Read the model definition and answer for the solid it produces. Units are mm, in the model's axes. Give positions to 0.01 mm unless a question says otherwise; leave off trailing zeros. Order: outer loops, then holes, each group sorted by start corner. A loop starts at its lowest first (then second) coordinate and runs counter-clockwise, first axis right, second up. Notation, with made-up numbers: (51, 39) - (82, 39) arc R13 ccw to (82, 55) - close; hole circle Ø9 at (56, 0). An arc over 180 degrees is marked (long way). Use a Markdown table: item, result. Add a question column.
1. Consider L1, parallel to X at y = 171, z = 9; L2, parallel to X at y = 271.5, z = 3.25; L3, parallel to Y at x = 145.5, z = 1.75. Determine where each line is inside the solid, lowest interval first.
2. A cutting plane is placed at A-A on y = 168. Determine the outline of the cut face in (x, z), and give its area (3 significant figures).
3. A cutting plane is placed at C-C on z = 1.5. State how many separate pieces and enclosed holes the cut face has, and give its area (3 significant figures).
4. Flat-ended cylindrical pins translate along their axes: P1, Ø3, axis at y = -192.5, z = 3, coming from the +X side; P2, Ø5, axis at x = -100, z = 5.5, coming from the -Y side; P3, Ø5, axis at x = 72, z = 3.5, coming from the +Y side; P4, Ø5, axis at x = 17, y = -29.5, coming from the -Z side. Find the tip coordinate at first contact, or state that the pin passes through.
5. A cutting plane is placed at B-B on y = 279. Determine the outline of the cut face in (x, z).
```python
from build123d import *

# Parameters (mm, degrees)
BOSS_EXTRU_1_DEPTH      = 10
ESQUISSE2_W             = 150
ESQUISSE2_H             = 120
BOSS_EXTRU_2_DEPTH      = 10
ESQUISSE3_W             = 10
ESQUISSE3_H             = 50
ESQUISSE3_W_2           = 50
ESQUISSE3_H_2           = 10
ENL_V_MAT_EXTRU_1_DEPTH = 10
ESQUISSE4_W             = 50
ESQUISSE4_H             = 10
ENL_V_MAT_EXTRU_2_DEPTH = 10


with BuildPart() as part:
    # Esquisse1 → Boss.-Extru.1 (new body)
    with BuildSketch(Plane.XY):
        Polygon((-50, 335.901139535), (50, 335.901139535), (255.775862069, 10.507079064), (205, -75.642859016), (-205, -75.642859016), (-255.775862069, 10.507079064), align=None)
        with BuildLine():
            Line((-189.319805153, 31.819805153), (-191.794678888, 34.294678888))
            ThreePointArc((-191.794678888, 34.294678888), (-206, 0), (-191.794678888, -34.294678888))
            Line((-191.794678888, -34.294678888), (-189.319805153, -31.819805153))
            ThreePointArc((-189.319805153, -31.819805153), (-202.5, 0), (-189.319805153, 31.819805153))
        make_face(mode=Mode.SUBTRACT)
        with BuildLine():
            Line((-125.680194847, 31.819805153), (-123.205321112, 34.294678888))
            ThreePointArc((-123.205321112, 34.294678888), (-109, 0), (-123.205321112, -34.294678888))
            Line((-123.205321112, -34.294678888), (-125.680194847, -31.819805153))
            ThreePointArc((-125.680194847, -31.819805153), (-112.5, 0), (-125.680194847, 31.819805153))
        make_face(mode=Mode.SUBTRACT)
        with BuildLine():
            Line((-84.319805153, -31.819805153), (-86.794678888, -34.294678888))
            ThreePointArc((-86.794678888, -34.294678888), (-101, 0), (-86.794678888, 34.294678888))
            Line((-86.794678888, 34.294678888), (-84.319805153, 31.819805153))
            ThreePointArc((-84.319805153, 31.819805153), (-97.5, 0), (-84.319805153, -31.819805153))
        make_face(mode=Mode.SUBTRACT)
        with BuildLine():
            Line((-20.680194847, 31.819805153), (-18.205321112, 34.294678888))
            ThreePointArc((-18.205321112, 34.294678888), (-4, 0), (-18.205321112, -34.294678888))
            Line((-18.205321112, -34.294678888), (-20.680194847, -31.819805153))
            ThreePointArc((-20.680194847, -31.819805153), (-7.5, 0), (-20.680194847, 31.819805153))
        make_face(mode=Mode.SUBTRACT)
        with BuildLine():
            Line((20.680194847, -31.819805153), (18.205321112, -34.294678888))
            ThreePointArc((18.205321112, -34.294678888), (4, 0), (18.205321112, 34.294678888))
            Line((18.205321112, 34.294678888), (20.680194847, 31.819805153))
            ThreePointArc((20.680194847, 31.819805153), (7.5, 0), (20.680194847, -31.819805153))
        make_face(mode=Mode.SUBTRACT)
        with BuildLine():
            Line((84.319805153, 31.819805153), (86.794678888, 34.294678888))
            ThreePointArc((86.794678888, 34.294678888), (101, 0), (86.794678888, -34.294678888))
            Line((86.794678888, -34.294678888), (84.319805153, -31.819805153))
            ThreePointArc((84.319805153, -31.819805153), (97.5, 0), (84.319805153, 31.819805153))
        make_face(mode=Mode.SUBTRACT)
        with BuildLine():
            Line((125.680194847, -31.819805153), (123.205321112, -34.294678888))
            ThreePointArc((123.205321112, -34.294678888), (109, 0), (123.205321112, 34.294678888))
            Line((123.205321112, 34.294678888), (125.680194847, 31.819805153))
            ThreePointArc((125.680194847, 31.819805153), (112.5, 0), (125.680194847, -31.819805153))
        make_face(mode=Mode.SUBTRACT)
        with BuildLine():
            Line((189.319805153, 31.819805153), (191.794678888, 34.294678888))
            ThreePointArc((191.794678888, 34.294678888), (206, 0), (191.794678888, -34.294678888))
            Line((191.794678888, -34.294678888), (189.319805153, -31.819805153))
            ThreePointArc((189.319805153, -31.819805153), (202.5, 0), (189.319805153, 31.819805153))
        make_face(mode=Mode.SUBTRACT)
        with BuildLine():
            Line((-139.294678888, 56.63798851), (-136.819805153, 59.112862244))
            ThreePointArc((-136.819805153, 59.112862244), (-150, 90.932667397), (-136.819805153, 122.752472551))
            Line((-136.819805153, 122.752472551), (-139.294678888, 125.227346285))
            ThreePointArc((-139.294678888, 125.227346285), (-153.5, 90.932667397), (-139.294678888, 56.63798851))
        make_face(mode=Mode.SUBTRACT)
        with BuildLine():
            Line((-70.705321112, 56.63798851), (-73.180194847, 59.112862244))
            ThreePointArc((-73.180194847, 59.112862244), (-60, 90.932667397), (-73.180194847, 122.752472551))
            Line((-73.180194847, 122.752472551), (-70.705321112, 125.227346285))
            ThreePointArc((-70.705321112, 125.227346285), (-56.5, 90.932667397), (-70.705321112, 56.63798851))
        make_face(mode=Mode.SUBTRACT)
        with BuildLine():
            Line((-31.819805153, 122.752472551), (-34.294678888, 125.227346285))
            ThreePointArc((-34.294678888, 125.227346285), (-48.5, 90.932667397), (-34.294678888, 56.63798851))
            Line((-34.294678888, 56.63798851), (-31.819805153, 59.112862244))
            ThreePointArc((-31.819805153, 59.112862244), (-45, 90.932667397), (-31.819805153, 122.752472551))
        make_face(mode=Mode.SUBTRACT)
        with BuildLine():
            Line((34.294678888, 56.63798851), (31.819805153, 59.112862244))
            ThreePointArc((31.819805153, 59.112862244), (45, 90.932667397), (31.819805153, 122.752472551))
            Line((31.819805153, 122.752472551), (34.294678888, 125.227346285))
            ThreePointArc((34.294678888, 125.227346285), (48.5, 90.932667397), (34.294678888, 56.63798851))
        make_face(mode=Mode.SUBTRACT)
        with BuildLine():
            Line((73.180194847, 122.752472551), (70.705321112, 125.227346285))
            ThreePointArc((70.705321112, 125.227346285), (56.5, 90.932667397), (70.705321112, 56.63798851))
            Line((70.705321112, 56.63798851), (73.180194847, 59.112862244))
            ThreePointArc((73.180194847, 59.112862244), (60, 90.932667397), (73.180194847, 122.752472551))
        make_face(mode=Mode.SUBTRACT)
        with BuildLine():
            Line((139.294678888, 56.63798851), (136.819805153, 59.112862244))
            ThreePointArc((136.819805153, 59.112862244), (150, 90.932667397), (136.819805153, 122.752472551))
            Line((136.819805153, 122.752472551), (139.294678888, 125.227346285))
            ThreePointArc((139.294678888, 125.227346285), (153.5, 90.932667397), (139.294678888, 56.63798851))
        make_face(mode=Mode.SUBTRACT)
        with BuildLine():
            Line((-84.319805153, 213.685139948), (-86.794678888, 216.160013682))
            ThreePointArc((-86.794678888, 216.160013682), (-101, 181.865334795), (-86.794678888, 147.570655907))
            Line((-86.794678888, 147.570655907), (-84.319805153, 150.045529641))
            ThreePointArc((-84.319805153, 150.045529641), (-97.5, 181.865334795), (-84.319805153, 213.685139948))
        make_face(mode=Mode.SUBTRACT)
        with BuildLine():
            Line((-20.680194847, 213.685139948), (-18.205321112, 216.160013682))
            ThreePointArc((-18.205321112, 216.160013682), (-4, 181.865334795), (-18.205321112, 147.570655907))
            Line((-18.205321112, 147.570655907), (-20.680194847, 150.045529641))
            ThreePointArc((-20.680194847, 150.045529641), (-7.5, 181.865334795), (-20.680194847, 213.685139948))
        make_face(mode=Mode.SUBTRACT)
        with BuildLine():
            Line((20.680194847, 150.045529641), (18.205321112, 147.570655907))
            ThreePointArc((18.205321112, 147.570655907), (4, 181.865334795), (18.205321112, 216.160013682))
            Line((18.205321112, 216.160013682), (20.680194847, 213.685139948))
            ThreePointArc((20.680194847, 213.685139948), (7.5, 181.865334795), (20.680194847, 150.045529641))
        make_face(mode=Mode.SUBTRACT)
        with BuildLine():
            Line((84.319805153, 150.045529641), (86.794678888, 147.570655907))
            ThreePointArc((86.794678888, 147.570655907), (101, 181.865334795), (86.794678888, 216.160013682))
            Line((86.794678888, 216.160013682), (84.319805153, 213.685139948))
            ThreePointArc((84.319805153, 213.685139948), (97.5, 181.865334795), (84.319805153, 150.045529641))
        make_face(mode=Mode.SUBTRACT)
        with BuildLine():
            Line((-31.819805153, 304.617807345), (-34.294678888, 307.09268108))
            ThreePointArc((-34.294678888, 307.09268108), (-48.5, 272.798002192), (-34.294678888, 238.503323305))
            Line((-34.294678888, 238.503323305), (-31.819805153, 240.978197039))
            ThreePointArc((-31.819805153, 240.978197039), (-45, 272.798002192), (-31.819805153, 304.617807345))
        make_face(mode=Mode.SUBTRACT)
        with BuildLine():
            Line((31.819805153, 304.617807345), (34.294678888, 307.09268108))
            ThreePointArc((34.294678888, 307.09268108), (48.5, 272.798002192), (34.294678888, 238.503323305))
            Line((34.294678888, 238.503323305), (31.819805153, 240.978197039))
            ThreePointArc((31.819805153, 240.978197039), (45, 272.798002192), (31.819805153, 304.617807345))
        make_face(mode=Mode.SUBTRACT)
    extrude(amount=BOSS_EXTRU_1_DEPTH)

    # Esquisse2 → Boss.-Extru.2 (add)
    with BuildSketch(Plane.XY.offset(10)):
        with Locations((0, -135.642859016)):
            Rectangle(ESQUISSE2_W, ESQUISSE2_H)
    extrude(amount=-BOSS_EXTRU_2_DEPTH)

    # Esquisse3 → Enlèv. mat.-Extru.1 (cut)
    with BuildSketch(Plane.XY.offset(10)):
        with Locations((-70, -135.642859016)):
            Rectangle(ESQUISSE3_W, ESQUISSE3_H)
        with Locations((0, -190.642859016)):
            Rectangle(ESQUISSE3_W_2, ESQUISSE3_H_2)
        with Locations((70, -135.642859016)):
            Rectangle(ESQUISSE3_W, ESQUISSE3_H)
    extrude(amount=-ENL_V_MAT_EXTRU_1_DEPTH, mode=Mode.SUBTRACT)

    # Esquisse4 → Enlèv. mat.-Extru.2 (cut)
    with BuildSketch(Plane.XY.offset(10)):
        with Locations((-140, -70.642859016)):
            Rectangle(ESQUISSE4_W, ESQUISSE4_H)
        Polygon((-217.693965517, -54.105374496), (-209.078971709, -49.027788289), (-234.466902744, -5.952819249), (-243.081896552, -11.030405456), align=None)
        Polygon((-229.051724138, 52.766047956), (-220.599930359, 47.42122037), (-167.151654497, 131.939158154), (-175.603448276, 137.283985741), align=None)
        Polygon((-68.272344153, 288.297343056), (-76.724137931, 293.642170642), (-130.172413793, 209.124232858), (-121.720620015, 203.779405271), align=None)
        with Locations((0, 330.901139535)):
            Rectangle(ESQUISSE4_W, ESQUISSE4_H)
        with Locations((140, -70.642859016)):
            Rectangle(ESQUISSE4_W, ESQUISSE4_H)
        Polygon((234.466902744, -5.952819249), (243.081896552, -11.030405456), (217.693965517, -54.105374496), (209.078971709, -49.027788289), align=None)
        Polygon((167.151654497, 131.939158154), (175.603448276, 137.283985741), (229.051724138, 52.766047956), (220.599930359, 47.42122037), align=None)
        Polygon((121.720620015, 203.779405271), (130.172413793, 209.124232858), (76.724137931, 293.642170642), (68.272344153, 288.297343056), align=None)
    extrude(amount=-ENL_V_MAT_EXTRU_2_DEPTH, mode=Mode.SUBTRACT)


solid = part.part
```
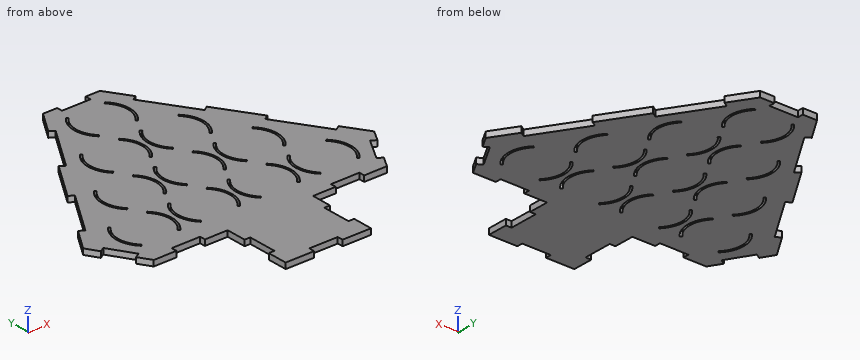
Output values:
| question | item | result |
|---|---|---|
| 1 | L1 | -154.28 to -99.77, -96.17 to -8.83, -5.23 to 5.23, 8.83 to 96.17, 99.77 to 154.28 |
| 1 | L2 | -78.89 to -48.48, -44.98 to 44.98, 48.48 to 78.89 |
| 1 | L3 | -65.64 to 64.25, 71.32 to 110.55, 117.62 to 184.89 |
| 2 | outline | (-156.18, 0) - (-98.98, 0) - (-98.98, 10) - (-156.18, 10) - close; (-95.31, 0) - (-9.69, 0) - (-9.69, 10) - (-95.31, 10) - close; (-6.02, 0) - (6.02, 0) - (6.02, 10) - (-6.02, 10) - close; (9.69, 0) - (95.31, 0) - (95.31, 10) - (9.69, 10) - close; (98.98, 0) - (156.18, 0) - (156.18, 10) - (98.98, 10) - close |
| 2 | area | 2,980 mm² |
| 3 | separate pieces | 1 |
| 3 | enclosed holes | 20 |
| 3 | area | 144,000 mm² |
| 4 | P1 | x = 75 |
| 4 | P2 | y = -75.64 |
| 4 | P3 | y = 305.07 |
| 4 | P4 | z = 0 |
| 5 | outline | (-74.15, 0) - (-48.1, 0) - (-48.1, 10) - (-74.15, 10) - close; (-44.57, 0) - (44.57, 0) - (44.57, 10) - (-44.57, 10) - close; (48.1, 0) - (74.15, 0) - (74.15, 10) - (48.1, 10) - close |
